Job drawing, mm, ordinate dimensions from the low corner. One solid piece. A direction names the side the tool comes from. Round coordinates to 2 decimals unless told otherwise and drop trailing zeros. Loops run counter-clockwise (first coordinate to the right, second up) from the corner with the lowest first, then second, coordinate; pieces in that order, holes last. Notation, with made-up numbers: M -18,1 L 30,1 A7 ccw 30,8 Z; hole C 21,27.5 d3. An arc over 180 degrees is marked long. One line per item, written item: value.
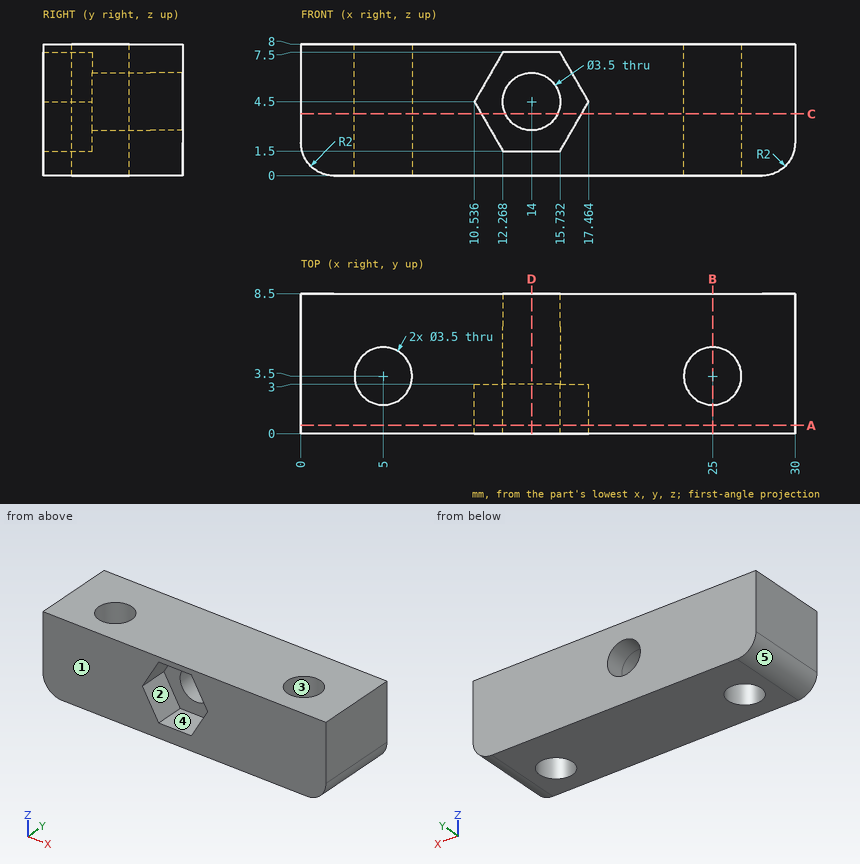
Item 1: Wall check: line 1 along Y through (x, z) = (5, 4); line 2 along X through (y, z) = (7.75, 4.5); line 3 along X through (y, z) = (4.8, 4.5). Give the ranges that are in metal, low to high.
Check values:
line 1: y = 0 to 1.75, 5.25 to 8.5
line 2: x = 0 to 12.25, 15.75 to 30
line 3: x = 0 to 3.83, 6.17 to 12.25, 15.75 to 23.83, 26.17 to 30
Item 2: Slice it at C-C, the plane z = 3.75. Give the cut face in (x, y).
Check values:
outline: M 0,0 L 10.97,0 L 10.97,3 L 12.42,3 L 12.42,8.5 L 0,8.5 Z; M 15.58,3 L 17.03,3 L 17.03,0 L 30,0 L 30,8.5 L 15.58,8.5 Z; hole C 5,3.5 d3.5; hole C 25,3.5 d3.5
Item 3: Pull direction Y, two halves, no side cores. Call the marked faces 1, 2 and 3: pulls with the +Y half, pulls with the -Y half, needs draft (parallel to the pull), parting line crosses it, or undercut.
Check values:
face 1: pulls with the -Y half
face 2: needs draft
face 3: undercut
Item 4: Slice it at A-A, the plane y = 0.5. Give the cut face in (x, z).
Check values:
outline: M 0,2 A2 ccw 2,0 L 28,0 A2 ccw 30,2 L 30,8 L 0,8 Z; hole M 10.54,4.5 L 12.27,1.5 L 15.73,1.5 L 17.46,4.5 L 15.73,7.5 L 12.27,7.5 Z
Item 5: Slice it at B-B, the plane x = 25. Give the cut face in (y, z), and give its area (3 significant figures).
Check values:
outline: M 0,0 L 1.75,0 L 1.75,8 L 0,8 Z; M 5.25,0 L 8.5,0 L 8.5,8 L 5.25,8 Z
area: 40.0 mm2
Item 6: Which spindle directions (+Z, -Z, +X, -X, +Y, -Y) get a long thin tool onto all of the face, cutting with end or side? Do the marked faces 4 and 5. Say none if no direction does.
Check values:
face 4: -Y
face 5: -Z, -X, +Y, -Y
Item 7: Slice it at D-D, the plane x = 14. Give the cut face in (y, z).
Check values:
outline: M 0,0 L 8.5,0 L 8.5,2.75 L 3,2.75 L 3,1.5 L 0,1.5 Z; M 0,7.5 L 3,7.5 L 3,6.25 L 8.5,6.25 L 8.5,8 L 0,8 Z
Item 8: Drop flat-ended pins along their axis: P1, Ø4, axis at x = 14, z = 4.5, coming from the -Y side; P2, Ø3, axis at x = 25, y = 3.5, coming from the -Z side. Give the stop position or say it passes through.
Check values:
P1: stops at y = 3
P2: passes through
